Could you check a few things on this model? Use its own coordinates, in mm. Round coordinates to 2 decimals unless told otherwise and drop trailing zeros. Order: outer loops, then holes, each group sorted by start corner. A loop starts at its lowest first (then second) coordinate and runs counter-clockwise, first axis right, second up. Notation, with made-up numbers: (73.25, 29) -> (96.25, 29) arc R24 cw to (96.25, 61) -> close; hole circle Ø6 at (6, 88). An arc over 180 degrees is marked (long way). One line per question, with ' | ' between items.
```python
from build123d import *

# Parameters (mm, degrees)
EXTRUDE_1_DEPTH     = 2
CUT_EXTRUDE_1_DEPTH = 1
CUT_EXTRUDE_2_DEPTH = 1
CUT_EXTRUDE_3_DEPTH = 3


with BuildPart() as part:
    # 스케치1 → 보스-돌출1 (new body)
    with BuildSketch(Plane(origin=(0, 0, 0), x_dir=(1, 0, 0), z_dir=(0, 1, 0))):
        Polygon((-33.25966317, -13.776603565), (-13.776603565, -33.25966317), (13.776603565, -33.25966317), (33.25966317, -13.776603565), (33.25966317, 13.776603565), (13.776603565, 33.25966317), (-13.776603565, 33.25966317), (-33.25966317, 13.776603565), align=None)
        Polygon((-13.27954729, -32.05966317), (13.27954729, -32.05966317), (32.05966317, -13.27954729), (32.05966317, 13.27954729), (13.27954729, 32.05966317), (-13.27954729, 32.05966317), (-32.05966317, 13.27954729), (-32.05966317, -13.27954729), align=None, mode=Mode.SUBTRACT)
        Polygon((-32.05966317, -13.27954729), (-13.27954729, -32.05966317), (13.27954729, -32.05966317), (32.05966317, -13.27954729), (32.05966317, 13.27954729), (13.27954729, 32.05966317), (-13.27954729, 32.05966317), (-32.05966317, 13.27954729), align=None)
    extrude(amount=EXTRUDE_1_DEPTH)

    # 스케치2 → 컷-돌출1 (cut)
    with BuildSketch(Plane(origin=(0, 2, 0), x_dir=(1, 0, 0), z_dir=(0, 1, 0))):
        Polygon((-32.05966317, -13.27954729), (-13.27954729, -32.05966317), (13.27954729, -32.05966317), (32.05966317, -13.27954729), (32.05966317, 13.27954729), (13.27954729, 32.05966317), (-13.27954729, 32.05966317), (-32.05966317, 13.27954729), align=None)
        Polygon((-30.85966317, -12.782491015), (-12.782491015, -30.85966317), (12.782491015, -30.85966317), (30.85966317, -12.782491015), (30.85966317, 12.782491015), (12.782491015, 30.85966317), (-12.782491015, 30.85966317), (-30.85966317, 12.782491015), align=None, mode=Mode.SUBTRACT)
    extrude(amount=-CUT_EXTRUDE_1_DEPTH, mode=Mode.SUBTRACT)

    # 스케치3 → 컷-돌출2 (cut)
    with BuildSketch(Plane(origin=(0, 2, 0), x_dir=(1, 0, 0), z_dir=(0, 1, 0))):
        Polygon((-14.320132754, -5.931593202), (-5.931593202, -14.320132754), (5.931593202, -14.320132754), (14.320132754, -5.931593202), (14.320132754, 5.931593202), (5.931593202, 14.320132754), (-5.931593202, 14.320132754), (-14.320132754, 5.931593202), align=None)
        Polygon((-5.434536927, -13.120132754), (5.434536927, -13.120132754), (13.120132754, -5.434536927), (13.120132754, 5.434536927), (5.434536927, 13.120132754), (-5.434536927, 13.120132754), (-13.120132754, 5.434536927), (-13.120132754, -5.434536927), align=None, mode=Mode.SUBTRACT)
    extrude(amount=-CUT_EXTRUDE_2_DEPTH, mode=Mode.SUBTRACT)

    # 스케치3<3> → 컷-돌출3 (cut)
    with BuildSketch(Plane(origin=(0, 2, 0), x_dir=(1, 0, 0), z_dir=(0, 1, 0))):
        Polygon((4.937480652, -11.920132754), (11.920132754, -4.937480652), (11.920132754, 4.937480652), (4.937480652, 11.920132754), (-4.937480652, 11.920132754), (-11.920132754, 4.937480652), (-11.920132754, -4.937480652), (-4.937480652, -11.920132754), align=None)
    extrude(amount=-CUT_EXTRUDE_3_DEPTH, mode=Mode.SUBTRACT)


solid = part.part
```
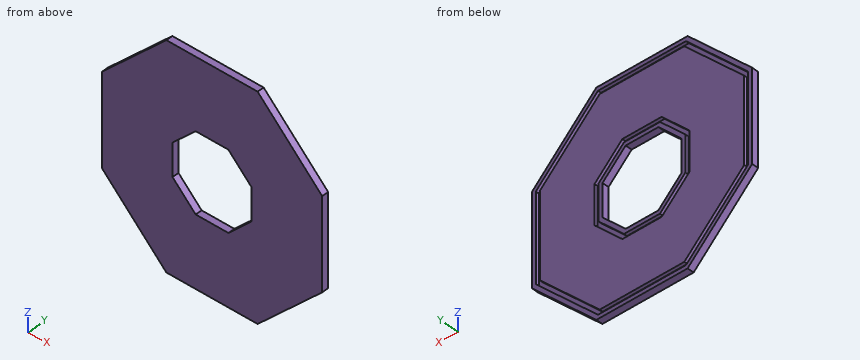
1. I'm going to push a flat-ended pin straight in: pin 1 (23 mm diameter, centred on x = 6, z = 0, fed in from +Y). Where does the tip first touch, or does it pass through?
From the geometry:
pin 1: stops at y = 2
2. I want a section at B-B on y = 1.45. Count the separate pieces of the cut face and the enclosed holes in it, and give its area (3 significant figures).
From the geometry:
separate pieces: 3 | enclosed holes: 3 | area: 2,840 mm²
3. I want a section at A-A on z = 4. List the corners of the cut face in (x, y) for me, and give its area (3 significant figures).
From the geometry:
outline: (-33.26, 0) -> (-11.92, 0) -> (-11.92, 2) -> (-13.12, 2) -> (-13.12, 1) -> (-14.32, 1) -> (-14.32, 2) -> (-30.86, 2) -> (-30.86, 1) -> (-32.06, 1) -> (-32.06, 2) -> (-33.26, 2) -> close; (11.92, 0) -> (33.26, 0) -> (33.26, 2) -> (32.06, 2) -> (32.06, 1) -> (30.86, 1) -> (30.86, 2) -> (14.32, 2) -> (14.32, 1) -> (13.12, 1) -> (13.12, 2) -> (11.92, 2) -> close | area: 80.6 mm²
4. I want a section at D-D on z = 25.5. List the corners of the cut face in (x, y) for me, and give its area (3 significant figures).
From the geometry:
outline: (-21.54, 0) -> (21.54, 0) -> (21.54, 2) -> (19.84, 2) -> (19.84, 1) -> (18.14, 1) -> (18.14, 2) -> (-18.14, 2) -> (-18.14, 1) -> (-19.84, 1) -> (-19.84, 2) -> (-21.54, 2) -> close | area: 82.8 mm²
5. I want a section at C-C on x = 17. List the corners of the cut face in (y, z) for me.
From the geometry:
outline: (0, -30.04) -> (2, -30.04) -> (2, -28.34) -> (1, -28.34) -> (1, -26.64) -> (2, -26.64) -> (2, 26.64) -> (1, 26.64) -> (1, 28.34) -> (2, 28.34) -> (2, 30.04) -> (0, 30.04) -> close
6. I need wall thicknesses on probe 1 along X at (y, z) = (1.55, 4.5); probe 2 along Z at (x, y) = (-15, 1.5). Which ranges of each line are inside material? Lowest first, please.
From the geometry:
probe 1: x = -33.26 to -32.06, -30.86 to -14.32, -13.12 to -11.92, 11.92 to 13.12, 14.32 to 30.86, 32.06 to 33.26 | probe 2: z = -32.04 to -30.34, -28.64 to 28.64, 30.34 to 32.04
